Geometry check sheet. Reference: the model listing, model coordinates, mm. Face numbers are marked on the shaded views. A direction names the side the tool comes from. Coordinates: 2 decimals unless noted, no trailing zeros. Order: outer loops, then holes, each group sorted by start corner. A loop starts at its lowest first (then second) coordinate and runs counter-clockwise, first axis right, second up. Notation, with made-up numbers: (-8.5, 0.25) - (23.5, 0.25) arc R18 cw to (23.5, 21.25) - close; hole circle Ø4 at (40.25, 37.25). An arc over 180 degrees is marked (long way). Return JSON: item names as keys, results as strings. Group by question number.
Item 1: Draft check along X on the marked faces 1, 2 and 3. Enter one of: pulls with the +X half, pulls with the -X half, needs draft (parallel to the pull), parting line crosses it, or undercut.
Item 2: Section check D-D on z = 192. Enter the section's corners in (x, y).
Item 3: Section check B-B on y = 22.5. Enter the section's corners in (x, z).
Item 4: Tool access check on the marked faces 4, 5 and 6. Record the directions out of +Z, -Z, +X, -X, +Y, -Y that give a thin tool (end or side, any length) a straight path to the whole face; none if there is none.
Item 5: Gauge pin test, flat ends, axial feed: pin 1 (3 mm diameter, centred on x = -27.5, z = 209, fed in from -Y); pin 2 (7.5 mm diameter, centred on y = 30, z = 240, fed in from +X); pin 3 (2 mm diameter, centred on x = 36, z = 120.5, fed in from +Y). Record the tip position at first contact, or that the pin passes through.
Item 6: Section check C-C on x = -18. Enter the section's corners in (y, z), then the cut area to 4 significant figures.
Item 7: Section check A-A on y = 67. Enter the section's corners in (x, z).
Item 8: Scan lines: probe 1 along Z at (x, y) = (-43, 104); probe 2 along X at (y, z) = (13, 114.5); probe 3 along Y at (x, z) = (4, 183). Record each from-to range of solid material in increasing order.
from build123d import *

# Parameters (mm, degrees)
SKETCH3_W           = 100
SKETCH3_H           = 7
BOSS_EXTRUDE3_DEPTH = 125
SKETCH4_W           = 100
SKETCH4_H           = 7
BOSS_EXTRUDE4_DEPTH = 140
CUT_EXTRUDE2_REACH  = 202.271
BOSS_EXTRUDE5_DEPTH = 7
BOSS_EXTRUDE6_DEPTH = 7
SKETCH8_W           = 100
SKETCH8_H           = 7
BOSS_EXTRUDE7_DEPTH = 120
SKETCH9_W           = 100
SKETCH9_H           = 7
BOSS_EXTRUDE8_DEPTH = 140
CUT_EXTRUDE3_REACH  = 292.703
SKETCH13_W          = 25
SKETCH13_H          = 64
CUT_EXTRUDE4_DEPTH  = 202.525034925
CHAMFER1_SIZE       = 10
CUT_EXTRUDE5_REACH  = 292.703
SKETCH15_W          = 25
SKETCH15_H          = 83


with BuildPart() as part:
    # Sketch3 → Boss-Extrude3 (new body)
    with BuildSketch(Plane.XY):
        with Locations((-3.612868806, 3.5)):
            Rectangle(SKETCH3_W, SKETCH3_H)
    extrude(amount=BOSS_EXTRUDE3_DEPTH)

    # Sketch4 → Boss-Extrude4 (add)
    with BuildSketch(Plane(origin=(0, 7, 0), x_dir=(1, 0, 0), z_dir=(0, 1, 0))):
        with Locations((-3.612868806, -121.5)):
            Rectangle(SKETCH4_W, SKETCH4_H)
    extrude(amount=BOSS_EXTRUDE4_DEPTH)

    # Sketch5 → Cut-Extrude2 (cut, up to next)
    with BuildSketch(Plane.XY.offset(125), mode=Mode.PRIVATE) as cut_extrude2_sk1:
        with BuildLine():
            ThreePointArc((2.387131194, 30), (1.673895268, 32.837274331), (-0.296244016, 35))
            Line((-0.296244016, 35), (-6.929493596, 35))
            ThreePointArc((-6.929493596, 35), (-9.612868806, 30), (-6.929493596, 25))
            Line((-6.929493596, 25), (-0.296244016, 25))
            ThreePointArc((-0.296244016, 25), (1.673895268, 27.162725669), (2.387131194, 30))
        make_face()
    cut_extrude2_tool1 = extrude(cut_extrude2_sk1.sketch, amount=-CUT_EXTRUDE2_REACH, mode=Mode.PRIVATE) & part.part
    add(cut_extrude2_tool1.solids().sort_by_distance((-3.612869, 30, 125))[0], mode=Mode.SUBTRACT)

    # Sketch6 → Boss-Extrude5 (add)
    with BuildSketch(Plane.ZY.offset(53.612868806)):
        Polygon((125, 0), (125, 90), (35, 0), align=None)
    extrude(amount=-BOSS_EXTRUDE5_DEPTH)

    # Sketch7 → Boss-Extrude6 (add)
    with BuildSketch(Plane(origin=(46.387131194, 0, 0), x_dir=(0, 0, -1), z_dir=(1, 0, 0))):
        Polygon((-125, 0), (-125, 90), (-35, 0), align=None)
    extrude(amount=-BOSS_EXTRUDE6_DEPTH)

    # Sketch8 → Boss-Extrude7 (add)
    with BuildSketch(Plane.XY.offset(125)):
        with Locations((-3.612868806, 143.5)):
            Rectangle(SKETCH8_W, SKETCH8_H)
    extrude(amount=BOSS_EXTRUDE7_DEPTH)

    # Sketch9 → Boss-Extrude8 (add)
    with BuildSketch(Plane.XZ.offset(-140)):
        with Locations((-3.612868806, 241.5)):
            Rectangle(SKETCH9_W, SKETCH9_H)
    extrude(amount=BOSS_EXTRUDE8_DEPTH)

    # Sketch10 → Cut-Extrude3 (cut, up to next)
    with BuildSketch(Plane.XY.offset(245), mode=Mode.PRIVATE) as cut_extrude3_sk1:
        with BuildLine():
            Line((-8.716428721, 35), (-8.716428721, 19))
            ThreePointArc((-8.716428721, 19), (-3.612868806, 13.896440085), (1.490691109, 19))
            Line((1.490691109, 19), (1.490691109, 35))
            ThreePointArc((1.490691109, 35), (-3.612868806, 40.103559915), (-8.716428721, 35))
        make_face()
    cut_extrude3_tool1 = extrude(cut_extrude3_sk1.sketch, amount=-CUT_EXTRUDE3_REACH, mode=Mode.PRIVATE) & part.part
    add(cut_extrude3_tool1.solids().sort_by_distance((-3.612869, 27, 245))[0], mode=Mode.SUBTRACT)

    # Sketch13 → Cut-Extrude4 (cut, through all)
    with BuildSketch(Plane(origin=(0, 0, 118), x_dir=(-1, 0, 0), z_dir=(0, 0, -1))):
        with Locations((-33.887131194, 115)):
            Rectangle(SKETCH13_W, SKETCH13_H)
    extrude(amount=-CUT_EXTRUDE4_DEPTH, mode=Mode.SUBTRACT)

    # Chamfer1
    chamfer1_edges = [part.edges().sort_by_distance(p)[0] for p in [
        (21.387131194, 83, 121.5),
    ]]
    chamfer(chamfer1_edges, length=CHAMFER1_SIZE)

    # Sketch15 → Cut-Extrude5 (cut, up to next)
    with BuildSketch(Plane.XY.offset(245), mode=Mode.PRIVATE) as cut_extrude5_sk1:
        with Locations((33.887131194, 41.5)):
            Rectangle(SKETCH15_W, SKETCH15_H)
    cut_extrude5_tool1 = extrude(cut_extrude5_sk1.sketch, amount=-CUT_EXTRUDE5_REACH, mode=Mode.PRIVATE) & part.part
    add(cut_extrude5_tool1.solids().sort_by_distance((33.887131, 41.5, 245))[0], mode=Mode.SUBTRACT)


solid = part.part
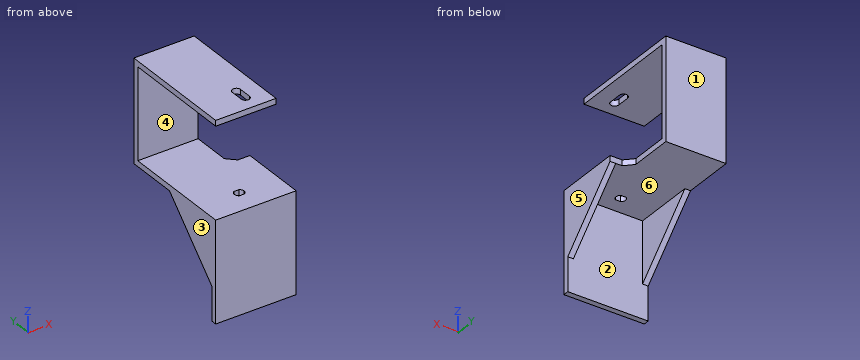
Computed:
{
 "1": {"face 1": "needs draft", "face 2": "undercut", "face 3": "pulls with the -X half"},
 "2": {"outline": "(-53.61, 140) - (21.39, 140) - (21.39, 147) - (-53.61, 147) - close"},
 "3": {"outline": "(-53.61, 57.5) - (-46.61, 57.5) - (-46.61, 118) - (39.39, 118) - (39.39, 57.5) - (46.39, 57.5) - (46.39, 125) - (-53.61, 125) - close; (-53.61, 238) - (-8.72, 238) - (-8.72, 245) - (-53.61, 245) - close; (1.49, 238) - (21.39, 238) - (21.39, 245) - (1.49, 245) - close"},
 "4": {"face 4": "+X, -X, -Y", "face 5": "+Z, -Z, +X, +Y, -Y", "face 6": "-Z, +Y"},
 "5": {"pin 1": "stops at y = 140", "pin 2": "stops at x = 21.39", "pin 3": "stops at y = 83"},
 "6": {"outline": "(0, 0) - (7, 0) - (7, 118) - (147, 118) - (147, 245) - (0, 245) - (0, 238) - (140, 238) - (140, 125) - (0, 125) - close", "area": "3,675 mm²"},
 "7": {"outline": "(-53.61, 102) - (-46.61, 102) - (-46.61, 118) - (39.39, 118) - (39.39, 102) - (46.39, 102) - (46.39, 125) - (-53.61, 125) - close; (-53.61, 238) - (21.39, 238) - (21.39, 245) - (-53.61, 245) - close"},
 "8": {"probe 1": "z = 118 to 125, 238 to 245", "probe 2": "x = -53.61 to -46.61, 39.39 to 46.39", "probe 3": "y = 140 to 147"}
}
